CAD build for the part. Positions are in the model's coordinates, mm. Face numbers are marked on the shaded views. A direction names the side the tool comes from. Round coordinates to 2 decimals unless told otherwise and drop trailing zeros. Write each loop counter-clockwise with the first axis right and the second up, starting at its lowest first coordinate (ties: lowest second). Pieces come first, ordered by that corner, then holes. Notation, with made-up numbers: (75, -35.5) -> (111, -35.5) arc R17 ccw to (111, -17.5) -> close; hole circle Ø5 at (30, 75.5). An arc over 180 degrees is marked (long way). Put each result on its own line as item: value. Start each with the question number.
1. Saw through at C-C on y = 13.75. List the corners of the cut face in (x, z), and give its area (3 significant figures).
2. Drill centre lines: line 1 (Y direction, x = 11.9, z = -9.85); line 2 (X direction, y = 2, z = -6.25); line 3 (X direction, y = 3.25, z = -3.9). Where is each one in solid material? Low to high. Write a range as from..to.
3. Pull direction Y, two halves, no side cores. Call the marked faces 1, 2 and 3: pulls with the +Y half, pulls with the -Y half, needs draft (parallel to the pull), parting line crosses it, or undercut.
4. Saw through at D-D on x = 7.9. List the corners of the cut face in (y, z), and give its area (3 significant figures).
5. 3-axis set-ups, long thin cutter, end or side, ignore diameter. For the marked faces 4, 5, 6, 7 and 8: which of +Z, -Z, +X, -X, +Y, -Y reach the whole face in a straight line?
6. Flat gauge pins, fed straight in: P1, Ø1.6, axis at x = 12, z = -4, coming from the -Y side; P2, Ø1.5, axis at x = 7.5, z = -4, coming from the -Y side; P3, Ø1, axis at x = 2, z = -6.5, coming from the +Y side. Where does each tip first touch, or does it go through?
from build123d import *

# Parameters (mm, degrees)
SKETCH1_W                 = 15.8
SKETCH1_H                 = 3.2
BOSS_EXTRUDE1_DEPTH       = 7.8
SKETCH2_R                 = 2.4
BOSS_EXTRUDE2_DEPTH       = 1.6
LPATTERN1_COUNT           = 2
LPATTERN1_PITCH           = 8
LPATTERN1_COUNT_DIR2      = 4
LPATTERN1_PITCH_DIR2      = 8
SHELL1_T                  = -0.8
SKETCH3_R                 = 1.5
SKETCH3_R_2               = 0.6
BOSS_EXTRUDE3_DEPTH       = 2.2
SKETCH4_W                 = 15.8
SKETCH4_H                 = 7.9
BOSS_EXTRUDE4_DEPTH       = 1.3
SKETCH5_R                 = 2.35
SKETCH5_R_2               = 1.65
BOSS_EXTRUDE5_DEPTH       = 1.6
LPATTERN2_COUNT           = 2
LPATTERN2_PITCH           = 8
SKETCH7_W                 = 1.1
SKETCH7_H                 = 2.4
BOSS_EXTRUDE6_DEPTH       = 0.5
LPATTERN3_COUNT           = 3
LPATTERN3_PITCH           = 4
SKETCH8_W                 = 15.8
SKETCH8_H                 = 1.3
BOSS_EXTRUDE7_DEPTH       = 7.9
MIRROR1_COPY_1_SKETCH_R   = 2.35
MIRROR1_COPY_1_SKETCH_R_2 = 1.65
MIRROR1_COPY_1_DEPTH      = 1.6
FILLET2_R                 = 0.5


with BuildPart() as part:
    # Sketch1 → Boss-Extrude1 (new body)
    with BuildSketch(Plane.XY):
        with Locations((7.9, 1.6)):
            Rectangle(SKETCH1_W, SKETCH1_H)
    extrude(amount=-BOSS_EXTRUDE1_DEPTH)

    # Sketch2 → Boss-Extrude2 (add)
    with BuildSketch(Plane(origin=(0, 3.2, 0), x_dir=(1, 0, 0), z_dir=(0, 1, 0))):
        with Locations(Location((3.9, 3.9, 0), (0, 0, 270))):
            Circle(SKETCH2_R)
    boss_extrude2 = extrude(amount=BOSS_EXTRUDE2_DEPTH)

    # LPattern1: Boss-Extrude2 2 × 4, 6 skipped
    with Locations(*[(j * LPATTERN1_PITCH_DIR2, 0, i * LPATTERN1_PITCH) for i in range(LPATTERN1_COUNT) for j in range(LPATTERN1_COUNT_DIR2) if (i, j) not in ((0, 0), (0, 2), (0, 3), (1, 0), (1, 1), (1, 2), (1, 3))]):
        add(boss_extrude2)

    # Shell1
    shell1_openings = [part.faces().sort_by_distance(p)[0] for p in [
        (7.9, 0, -3.9),
    ]]
    offset(amount=SHELL1_T, openings=shell1_openings, kind=Kind.INTERSECTION)

    # Sketch3 → Boss-Extrude3 (add)
    with BuildSketch(Plane.XZ.offset(-2.4)):
        with Locations(Location((7.9, -3.9, 0), (0, 0, 90))):
            Circle(SKETCH3_R)
        with Locations(Location((7.9, -3.9, 0), (0, 0, 270))):
            Circle(SKETCH3_R_2, mode=Mode.SUBTRACT)
    extrude(amount=BOSS_EXTRUDE3_DEPTH)

    # Sketch4 → Boss-Extrude4 (add)
    with BuildSketch(Plane(origin=(0, 0, -7.8), x_dir=(-1, 0, 0), z_dir=(0, 0, -1))):
        with Locations((-7.9, 3.95)):
            Rectangle(SKETCH4_W, SKETCH4_H)
    extrude(amount=BOSS_EXTRUDE4_DEPTH)

    # Sketch5 → Boss-Extrude5 (add)
    with BuildSketch(Plane(origin=(0, 0, -9.1), x_dir=(-1, 0, 0), z_dir=(0, 0, -1))):
        with Locations(Location((-11.9, 4, 0), (0, 0, 180))):
            Circle(SKETCH5_R)
        with Locations((-11.9, 4)):
            Circle(SKETCH5_R_2, mode=Mode.SUBTRACT)
    boss_extrude5 = extrude(amount=BOSS_EXTRUDE5_DEPTH)

    # LPattern2: Boss-Extrude5 ×2
    with Locations(*[(-i * LPATTERN2_PITCH, 0, 0) for i in range(1, LPATTERN2_COUNT)]):
        add(boss_extrude5)

    # Sketch7 → Boss-Extrude6 (add)
    with BuildSketch(Plane.XY.offset(-7)):
        with Locations((11.9, 1.2)):
            Rectangle(SKETCH7_W, SKETCH7_H)
    boss_extrude6 = extrude(amount=BOSS_EXTRUDE6_DEPTH)

    # LPattern3: Boss-Extrude6 ×3
    with Locations(*[(-i * LPATTERN3_PITCH, 0, 0) for i in range(1, LPATTERN3_COUNT)]):
        add(boss_extrude6)

    # Sketch8 → Boss-Extrude7 (add)
    with BuildSketch(Plane(origin=(0, 7.9, 0), x_dir=(1, 0, 0), z_dir=(0, 1, 0))):
        with Locations((7.9, 8.45)):
            Rectangle(SKETCH8_W, SKETCH8_H)
    extrude(amount=BOSS_EXTRUDE7_DEPTH)

    # Mirror1: Boss-Extrude5 across plane
    add(boss_extrude5.mirror(Plane.ZX.offset(7.9)))

    # Mirror1 copy 1 sketch → Mirror1 copy 1 (add)
    with BuildSketch(Plane(origin=(-8, 15.8, -9.1), x_dir=(-1, 0, 0), z_dir=(0, 0, -1))):
        with Locations((-11.9, -4)):
            Circle(MIRROR1_COPY_1_SKETCH_R)
        with Locations((-11.9, -4)):
            Circle(MIRROR1_COPY_1_SKETCH_R_2, mode=Mode.SUBTRACT)
    extrude(amount=MIRROR1_COPY_1_DEPTH)

    # Fillet2
    fillet2_edges = [part.edges().sort_by_distance(p)[0] for p in [
        (0, 15.8, -8.45),
        (15.8, 15.8, -8.45),
    ]]
    fillet(fillet2_edges, radius=FILLET2_R)


solid = part.part
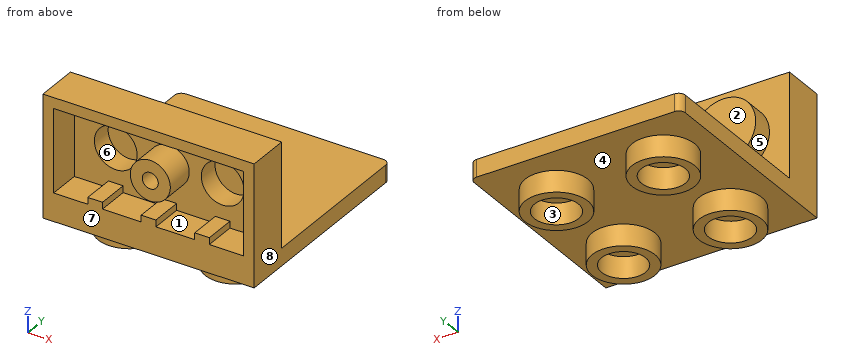
Return value:
1. outline: (0, -9.1) -> (2.59, -9.1) -> (2.59, -10.7) -> (5.21, -10.7) -> (5.21, -9.1) -> (10.59, -9.1) -> (10.59, -10.7) -> (13.21, -10.7) -> (13.21, -9.1) -> (15.8, -9.1) -> (15.8, -7.8) -> (0, -7.8) -> close
1. area: 28.9 mm^2
2. line 1: y = 1.65..2.35, 5.65..6.35, 9.45..10.15, 13.45..14.15
2. line 2: x = 0..0.8, 15..15.8
2. line 3: x = 1.5..2.3, 5.5..6.3, 9.5..10.3, 13.5..14.3
3. face 1: needs draft
3. face 2: pulls with the +Y half
3. face 3: undercut
4. outline: (0, -9.1) -> (15.8, -9.1) -> (15.8, -7.8) -> (3.2, -7.8) -> (3.2, 0) -> (0, 0) -> (0, -0.8) -> (2.4, -0.8) -> (2.4, -2.4) -> (0.2, -2.4) -> (0.2, -3.3) -> (2.4, -3.3) -> (2.4, -4.5) -> (0.2, -4.5) -> (0.2, -5.4) -> (2.4, -5.4) -> (2.4, -6.5) -> (0, -6.5) -> close
4. area: 35.8 mm^2
5. face 4: -Z
5. face 5: +Y
5. face 6: -Y
5. face 7: +Z, -Z, +X, -X, -Y
5. face 8: +Z, -Z, +X, +Y, -Y
6. P1: stops at y = 4
6. P2: stops at y = 0.2
6. P3: stops at y = 3.2
